Input: part model. Units: mm. Frame: model coordinates. A direction names the side the tool comes from. Coordinates: 2 decimals unless noted, no trailing zeros. Order: outer loops, then holes, each group sorted by start corner. A loop starts at its lowest first (then second) coordinate and runs counter-clockwise, first axis right, second up.
from build123d import *

# Parameters (mm, degrees)
BOSS_EXTRUDE1_DEPTH = 4.7625
CUT_EXTRUDE1_DEPTH  = 4.7625


with BuildPart() as part:
    # Sketch1 → Boss-Extrude1 (new body)
    with BuildSketch(Plane.XY):
        with BuildLine():
            Line((0, 21.034375), (8.436280557, 23.284685407))
            Line((8.436280557, 23.284685407), (9.663722597, 18.68307783))
            ThreePointArc((9.663722597, 18.68307783), (9.719485393, 18.654129176), (9.775161472, 18.62501409))
            Line((9.775161472, 18.62501409), (18.290888316, 16.697029938))
            Line((18.290888316, 16.697029938), (17.239260597, 12.052088023))
            ThreePointArc((17.239260597, 12.052088023), (17.27518299, 12.000541), (17.310951254, 11.948886907))
            Line((17.310951254, 11.948886907), (23.95527399, 6.284286132))
            Line((23.95527399, 6.284286132), (20.865491749, 2.660110094))
            ThreePointArc((20.865491749, 2.660110094), (20.873344353, 2.597773503), (20.881010724, 2.535413734))
            Line((20.881010724, 2.535413734), (24.131795086, -5.568111894))
            Line((24.131795086, -5.568111894), (19.711690198, -7.341267))
            ThreePointArc((19.711690198, -7.341267), (19.689674075, -7.400112598), (19.66748228, -7.458892171))
            Line((19.66748228, -7.458892171), (18.780012747, -16.144922587))
            Line((18.780012747, -16.144922587), (14.042177975, -15.660848297))
            ThreePointArc((14.042177975, -15.660848297), (13.995336753, -15.702722083), (13.948370664, -15.744455769))
            Line((13.948370664, -15.744455769), (9.125955812, -23.023126083))
            Line((9.125955812, -23.023126083), (5.155772004, -20.392717982))
            ThreePointArc((5.155772004, -20.392717982), (5.094836443, -20.408027177), (5.033855426, -20.423154291))
            Line((5.033855426, -20.423154291), (-2.61874762, -24.627008853))
            Line((-2.61874762, -24.627008853), (-4.9117592, -20.452861736))
            ThreePointArc((-4.9117592, -20.452861736), (-4.972829497, -20.438099188), (-5.033855426, -20.423154291))
            Line((-5.033855426, -20.423154291), (-13.763527532, -20.589140681))
            Line((-13.763527532, -20.589140681), (-13.854065563, -15.827501351))
            ThreePointArc((-13.854065563, -15.827501351), (-13.901280128, -15.786048982), (-13.948370664, -15.744455769))
            Line((-13.948370664, -15.744455769), (-21.755249155, -11.834548506))
            Line((-21.755249155, -11.834548506), (-19.622572466, -7.576251148))
            ThreePointArc((-19.622572466, -7.576251148), (-19.64511501, -7.517605196), (-19.66748228, -7.458892171))
            Line((-19.66748228, -7.458892171), (-24.763105375, -0.36880389))
            Line((-24.763105375, -0.36880389), (-20.895784495, 2.410626889))
            ThreePointArc((-20.895784495, 2.410626889), (-20.888490793, 2.473031344), (-20.881010724, 2.535413734))
            Line((-20.881010724, 2.535413734), (-22.098032582, 11.181429253))
            Line((-22.098032582, 11.181429253), (-17.382024117, 11.845259357))
            ThreePointArc((-17.382024117, 11.845259357), (-17.346565069, 11.897126206), (-17.310951254, 11.948886907))
            Line((-17.310951254, 11.948886907), (-14.370566834, 20.170131705))
            Line((-14.370566834, 20.170131705), (-9.88625149, 18.566285658))
            ThreePointArc((-9.88625149, 18.566285658), (-9.830750336, 18.59573283), (-9.775161472, 18.62501409))
            Line((-9.775161472, 18.62501409), (-3.350977409, 24.53810006))
            Line((-3.350977409, 24.53810006), (-0.125657789, 21.033999662))
            ThreePointArc((-0.125657789, 21.033999662), (-0.062829175, 21.034281165), (0, 21.034375))
        make_face()
    extrude(amount=BOSS_EXTRUDE1_DEPTH)

    # Sketch2 → Cut-Extrude1 (cut)
    with BuildSketch(Plane(origin=(0, 0, 0), x_dir=(-1, 0, 0), z_dir=(0, 0, -1))):
        Polygon((-7.332348419, 0), (-3.666174209, -6.35), (3.666174209, -6.35), (7.332348419, 0), (3.666174209, 6.35), (-3.666174209, 6.35), align=None)
    extrude(amount=-CUT_EXTRUDE1_DEPTH, mode=Mode.SUBTRACT)


solid = part.part
Item 1: Cut plane B-B on y = 4. Return loops of the section in (x, z), then the cut area to 3 significant figures.
Response values:
outline: (-21.09, 0) - (-5.02, 0) - (-5.02, 4.76) - (-21.09, 4.76) - close; (5.02, 0) - (22.01, 0) - (22.01, 4.76) - (5.02, 4.76) - close
area: 157 mm2
Item 2: Cut plane C-C on y = 18. Return loops of the section in (x, z).
Response values:
outline: (-15.15, 0) - (12.54, 0) - (12.54, 4.76) - (-15.15, 4.76) - close
Item 3: Access query for faces 1 (the face through (13.973, 17.675, 2.348)), 2 (the face through (-12.16, 19.38, 2.35)), 3 (the face through (1.261, -22.496, 2.348)), 4 (the face through (5.525, -3.131, 2.348)), 5 (the face through (-22.18, -3.96, 2.35)). Directions: +Z, -Z, +X, -X, +Y, -Y. A direction counts if a zero-diameter tool reaches every point of the face in a straight line with its end or side. Return the directions, or none.
Response values:
face 1: +Z, -Z, +X, +Y
face 2: +Z, -Z, +Y
face 3: +Z, -Z, -Y
face 4: +Z, -Z
face 5: +Z, -Z, -X
Item 4: Ray query, probe 1 along Y at (x, z) = (7, 4.55); probe 2 along Y at (x, z) = (-1.5, 0.65); probe 3 along X at (y, z) = (1, 1.1) (3 decimals). Return the intervals inside material, ascending.
Response values:
probe 1: y = -21.61 to -0.58, 0.58 to 22.9
probe 2: y = -24.01 to -6.35, 6.35 to 22.53
probe 3: x = -22.859 to -6.755, 6.755 to 21.497
Item 5: Cut plane A-A on x = -1. Return loops of the section in (y, z), then the cut area to 3 significant figures.
Response values:
outline: (-23.74, 0) - (-6.35, 0) - (-6.35, 4.76) - (-23.74, 4.76) - close; (6.35, 0) - (21.98, 0) - (21.98, 4.76) - (6.35, 4.76) - close
area: 157 mm2
Item 6: Cut plane D-D on x = -8. Return loops of the section in (y, z), then the cut area to 3 significant figures.
Response values:
outline: (-20.48, 0) - (20.26, 0) - (20.26, 4.76) - (-20.48, 4.76) - close
area: 194 mm2
Item 7: Pin query (flat end, axial travel): pin 1 Ø8 at (x, y) = (-19.5, -10) entering from -Z; pin 2 Ø1 at (x, y) = (4.5, 1) entering from +Z; pin 3 Ø1 at (y, z) = (7.5, 2) entering from -X. Return the tip coordinate at first contact, or that it passes through.
Response values:
pin 1: stops at z = 0
pin 2: passes through
pin 3: stops at x = -21.65
Item 8: Draft query along X for faces 6 (the face through (-15.86, 16, 2.35)), 7 (the face through (19.23, -11.74, 2.35)), 8 (the face through (5, 6, 4.762)), 9 (the face through (-6.61, 21.54, 2.35)). Return one class per face: pulls with the +X half, pulls with the -X half, needs draft (parallel to the pull), parting line crosses it, or undercut.
Response values:
face 6: pulls with the -X half
face 7: pulls with the +X half
face 8: needs draft
face 9: undercut
